Autodesk Inventor part; units mm, degrees
ref_plane "YZ Plane" through (0, 0, 0) normal (1, 0, 0) x (0, 1, 0)
ref_plane "XZ Plane" through (0, 0, 0) normal (0, 1, 0) x (-1, 0, 0)
ref_plane "XY Plane" through (0, 0, 0) normal (0, 0, 1) x (1, 0, 0)
sketch "草圖1" plane through (0, 0, 0) normal (0, 1, 0) x (-1, 0, 0)
  line L0 (0, -20) -> (-40, -20)
  line L1 (-40, -20) -> (-40, 20)
  line L2 (-40, 20) -> (0, 20)
  line L3 (0, 20) -> (0, -20)
  point P0 (0, 0)
  point P1 (0, 0)
  dimension "d0" = 40
  dimension "d1" = 40
extrude "擠出1" add sketch "草圖1" along normal blind 20
sketch "草圖2" plane through (0, 20, 0) normal (0, 1, 0) x (1, 0, 0)
  line L0 (0, 20) -> (40, 20)
  line L1 (40, 20) -> (40, -20)
  line L2 (40, -20) -> (0, -20)
  line L3 (0, -20) -> (0, 20)
  line L4 (10, 10) -> (40, 10)
  line L5 (40, 10) -> (40, -10)
  line L6 (40, -10) -> (10, -10)
  line L7 (10, -10) -> (10, 10)
  point P0 (0, 0)
  point P1 (40, 0)
  dimension "d4" = 20
  dimension "d5" = 30
extrude "擠出2" cut sketch "草圖2" against normal through all contours L1 L6 L7 L4
sketch "草圖3" plane through (0, 0, 20) normal (0, 0, 1) x (1, 0, 0)
  line L0 (40, 0) -> (0, 0)
  line L1 (0, 0) -> (0, 20)
  line L2 (0, 20) -> (40, 20)
  line L3 (40, 20) -> (40, 0)
  line L4 (40, 0) -> (40, 20)
  line L5 (40, 0) -> (20, 20)
  dimension "d8" = 20
extrude "擠出3" cut sketch "草圖3" against normal blind 13 contours L5 L2 L3
sketch "草圖4" plane through (10, 20, -10) normal (0, 0, 1) x (1, 0, 0)
  line L0 (-10, 0) -> (0, 0)
  line L1 (0, 0) -> (30, 0)
  line L2 (30, 0) -> (30, -20)
  line L3 (30, -20) -> (0, -20)
  line L4 (0, -20) -> (-10, -20)
  line L5 (-10, -20) -> (-10, 0)
  line L6 (0, 0) -> (0, -20)
  line L7 (0, 0) -> (20, -20)
  line L8 (30, -20) -> (-10, -20)
  dimension "d11" = 30
extrude "擠出4" add sketch "草圖4" along normal up to surface (20 mm away) contours L7 L3 L6
properties part number "48" material "鋼、碳鋼"
Check sheet for the modelled part. Datum: model origin and axes. Units: mm. A direction names the side the tool comes from. Round coordinates to 2 decimals unless told otherwise and drop trailing zeros. Order: outer loops, then holes, each group sorted by start corner. A loop starts at its lowest first (then second) coordinate and runs counter-clockwise, first axis right, second up.
1) Section check C-C (x = 19). Record the boundary of the cut face in (y, z).
2) Scan lines: line 1 (Z direction, x = 24, y = 8.25); line 2 (Z direction, x = 36, y = 4.75); line 3 (X direction, y = 10, z = -4.5). Record each from-to range of solid material in increasing order.
3) Section check B-B (y = 16). Record the boundary of the cut face in (x, z), and give its area (3 significant figures).
4) Section check A-A (x = 37). Record the boundary of the cut face in (y, z).
5) Go/stop test with flat-tipped pins: pin 1 Ø4 at (y, z) = (9.5, 12) entering from +X; pin 2 Ø1 at (y, z) = (3, 7.5) entering from +X. Record where each tip stops, or that it passes through.
6) Section check D-D (z = -1). Record the boundary of the cut face in (x, y), and give its area (3 significant figures).
7) Mould release check, pull along Z, two halves, no side actions. Record for faces 1 (the flat face through (7, 20, -4)), 2 (the flat face through (28, 12, -10)), 3 (the flat face through (20, 10, -20)): +Z half, -Z half, draft (parallel to the pull), parting line (faces both ways), or undercut.
8) Tool access check on faces 4 (the flat face through (40, 10, -15)), 5 (the flat face through (25, 11, 10)), 6 (the flat face through (30, 10, 15)). Record the directions out of +Z, -Z, +X, -X, +Y, -Y that give a thin tool (end or side, any length) a straight path to the whole face; none if there is none.
Result:
1. outline: (0, -20) - (20, -20) - (20, -10) - (11, -10) - (11, 10) - (20, 10) - (20, 20) - (0, 20) - close
2. line 1: z = -20 to -10, 10 to 20
2. line 2: z = -20 to -10
2. line 3: x = 0 to 20
3. outline: (0, -20) - (40, -20) - (40, -10) - (14, -10) - (14, 10) - (24, 10) - (24, 20) - (0, 20) - close
3. area: 920 mm2
4. outline: (0, -20) - (20, -20) - (20, -10) - (0, -10) - close; (0, 10) - (3, 10) - (3, 20) - (0, 20) - close
5. pin 1: stops at x = 32.5
5. pin 2: stops at x = 27.5
6. outline: (0, 0) - (30, 0) - (10, 20) - (0, 20) - close
6. area: 400 mm2
7. face 1: draft
7. face 2: undercut
7. face 3: -Z half
8. face 4: +Z, -Z, +X, +Y, -Y
8. face 5: +X, +Y
8. face 6: +Z, +X, +Y
